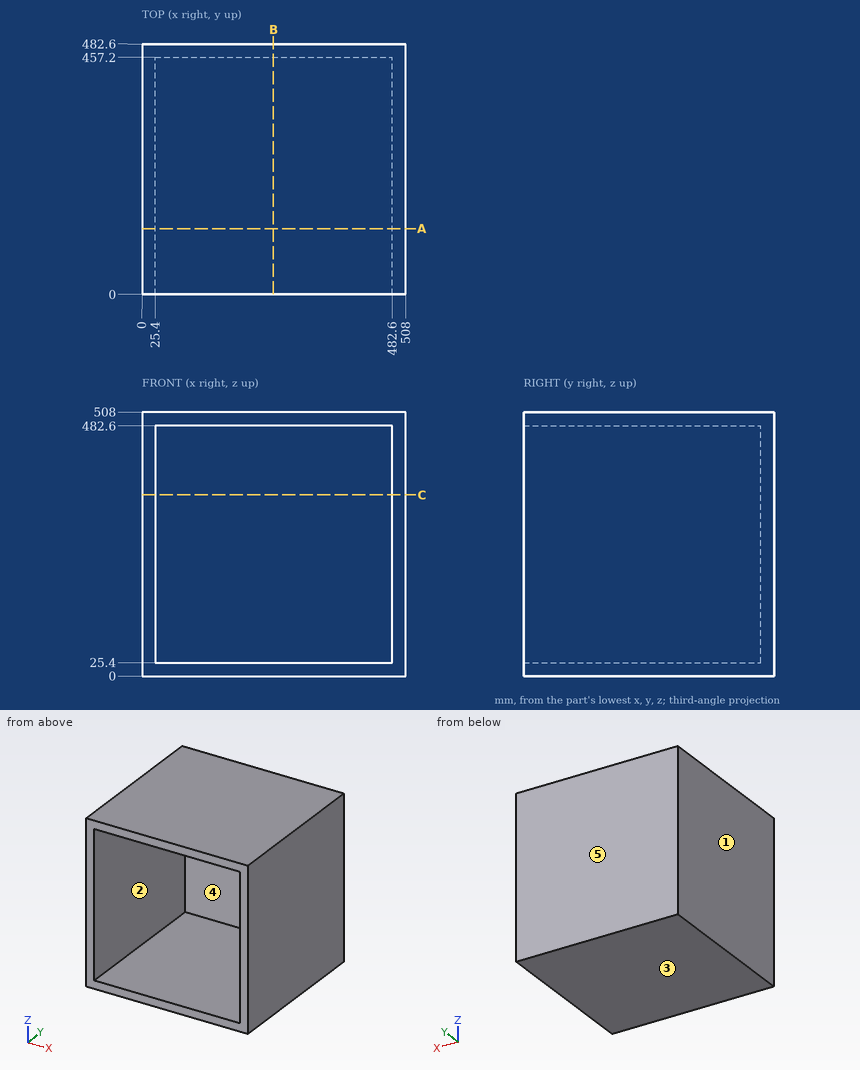
Geometry check sheet. Reference: drawing and pictorial views, mm from the part's lowest x, y, z. A direction names the side the tool comes from. Give positions to 0.01 mm unless a question says otherwise; leave off trailing zeros. Write each loop counter-clockwise with the first axis right and the second up, starting at its lowest first coordinate (ties: lowest second). Pieces come first, ordered by that corner, then holes. Notation, with made-up numbers: M -18,48.5 L 33,48.5 A33 ccw 33,81.5 Z; hole C 52.25,-8.5 d7. An arc over 180 degrees is marked long. Put each result on its own line as item: value. Start each with the question number.
1. Go/stop test with a flat-tipped pin: pin 1 Ø8 at (x, z) = (314.5, 101.5) entering from -Y. Record where the tip stops, or that it passes through.
2. Draft check along X on the marked faces 1, 2 and 3. Enter one of: +X half, -X half, draft (parallel to the pull), parting line (faces both ways), or undercut.
3. Section check B-B (x = 253). Record the cut outline in (y, z).
4. Scan lines: line 1 along Z through (x, y) = (233.5, 256); line 2 along Y through (x, z) = (134, 298.5). Record each from-to range of solid material in increasing order. Write a range as [from, to].
5. Set-up check for the marked faces 4 and 5: record each of +Z, -Z, +X, -X, +Y, -Y from which the full face is reachable in a straight line by a thin tool's end or side.
6. Section check A-A (y = 127). Record the cut outline in (x, z).
7. Section check C-C (z = 349). Record the cut outline in (x, y), and give its area (3 significant figures).
Answer list:
1. pin 1: y = 457.2
2. face 1: -X half
2. face 2: undercut
2. face 3: draft
3. outline: M 0,0 L 482.6,0 L 482.6,508 L 0,508 L 0,482.6 L 457.2,482.6 L 457.2,25.4 L 0,25.4 Z
4. line 1: [0, 25.4], [482.6, 508]
4. line 2: [457.2, 482.6]
5. face 4: -Y
5. face 5: +Z, -Z, +X, -X, +Y
6. outline: M 0,0 L 508,0 L 508,508 L 0,508 Z; hole M 25.4,25.4 L 482.6,25.4 L 482.6,482.6 L 25.4,482.6 Z
7. outline: M 0,0 L 25.4,0 L 25.4,457.2 L 482.6,457.2 L 482.6,0 L 508,0 L 508,482.6 L 0,482.6 Z
7. area: 36,100 mm2
